Could you check a few things on this drawing? It's one solid part, dimensions in mm from its lowest x, y, z. A direction names the side the tool comes from. Give positions to 0.01 mm unless a question says otherwise; leave off trailing zeros. Order: outer loops, then holes, each group sorted by start corner. A loop starts at its lowest first (then second) coordinate and runs counter-clockwise, first axis right, second up.
Item 1: If I drill on line 1 along X through (y, z) = (170, 40.5) (3 decimals); line 2 along Z through (x, y) = (5.75, 186) (3 decimals); line 3 along Y through (x, z) = (14, 3), over which ranges is the centre line in solid material (lowest first)?
Item 2: I want a section at C-C, the plane z = 13. Write out the boundary of the cut face in (x, y) (3 decimals).
Item 3: I want a section at B-B, the plane y = 156.5. Write out the boundary of the cut face in (x, z) (3 decimals).
Item 4: Which directions (+Z, -Z, +X, -X, +Y, -Y) give clear straight access to the entire face, cutting with the end or side of a thin tool? Please do the marked faces 1 and 2.
Item 5: If we mould it in two halves opening along X, with no side actions, what happens to the marked faces 3, 4 and 5? For each: +X half, -X half, draft (parallel to the pull), parting line (faces both ways), or undercut.
Item 6: I want a section at A-A, the plane x = 8. Write out the boundary of the cut face in (y, z) (3 decimals).
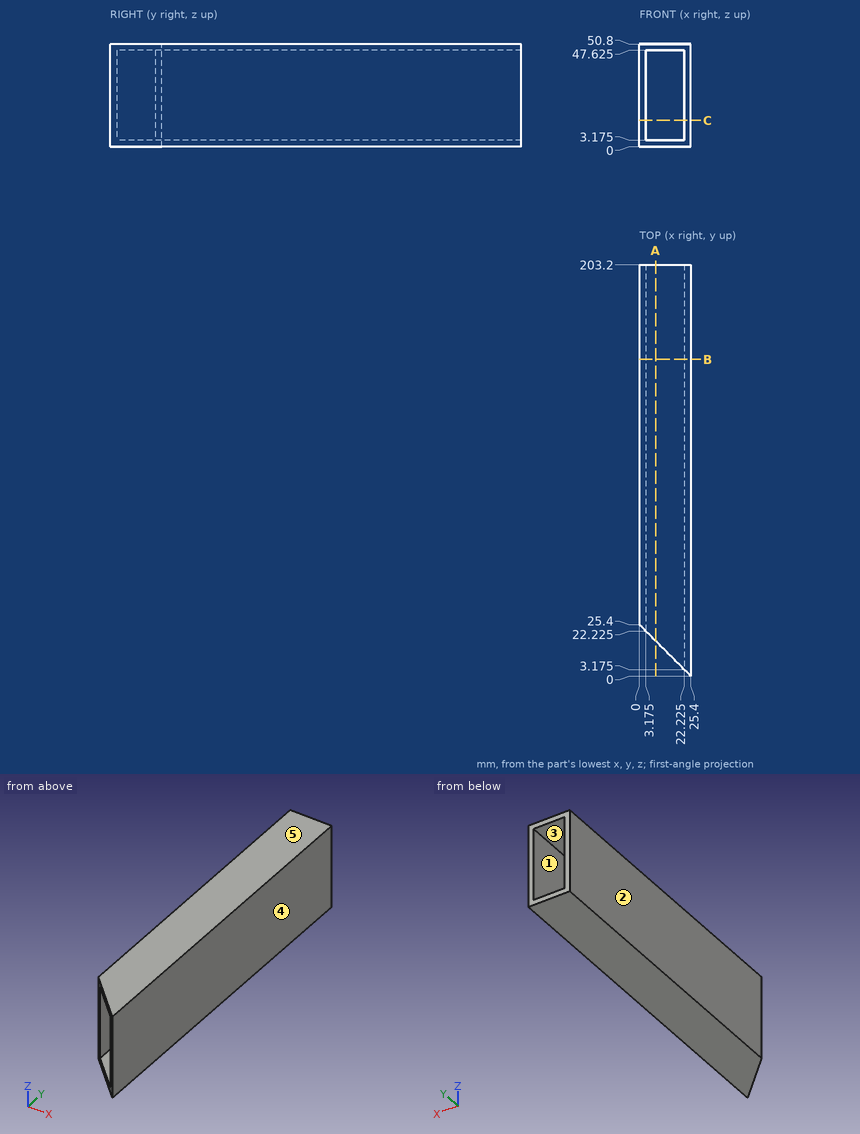
Results list:
1. line 1: x = 0 to 3.175, 22.225 to 25.4
1. line 2: z = 0 to 3.175, 47.625 to 50.8
1. line 3: y = 11.4 to 203.2
2. outline: (0, 25.4) - (3.175, 22.225) - (3.175, 203.2) - (0, 203.2) - close; (22.225, 3.175) - (25.4, 0) - (25.4, 203.2) - (22.225, 203.2) - close
3. outline: (0, 0) - (25.4, 0) - (25.4, 50.8) - (0, 50.8) - close; hole (3.175, 3.175) - (22.225, 3.175) - (22.225, 47.625) - (3.175, 47.625) - close
4. face 1: +Y, -Y
4. face 2: +Z, -Z, -X, +Y, -Y
5. face 3: undercut
5. face 4: +X half
5. face 5: draft
6. outline: (17.4, 0) - (203.2, 0) - (203.2, 3.175) - (17.4, 3.175) - close; (17.4, 47.625) - (203.2, 47.625) - (203.2, 50.8) - (17.4, 50.8) - close
